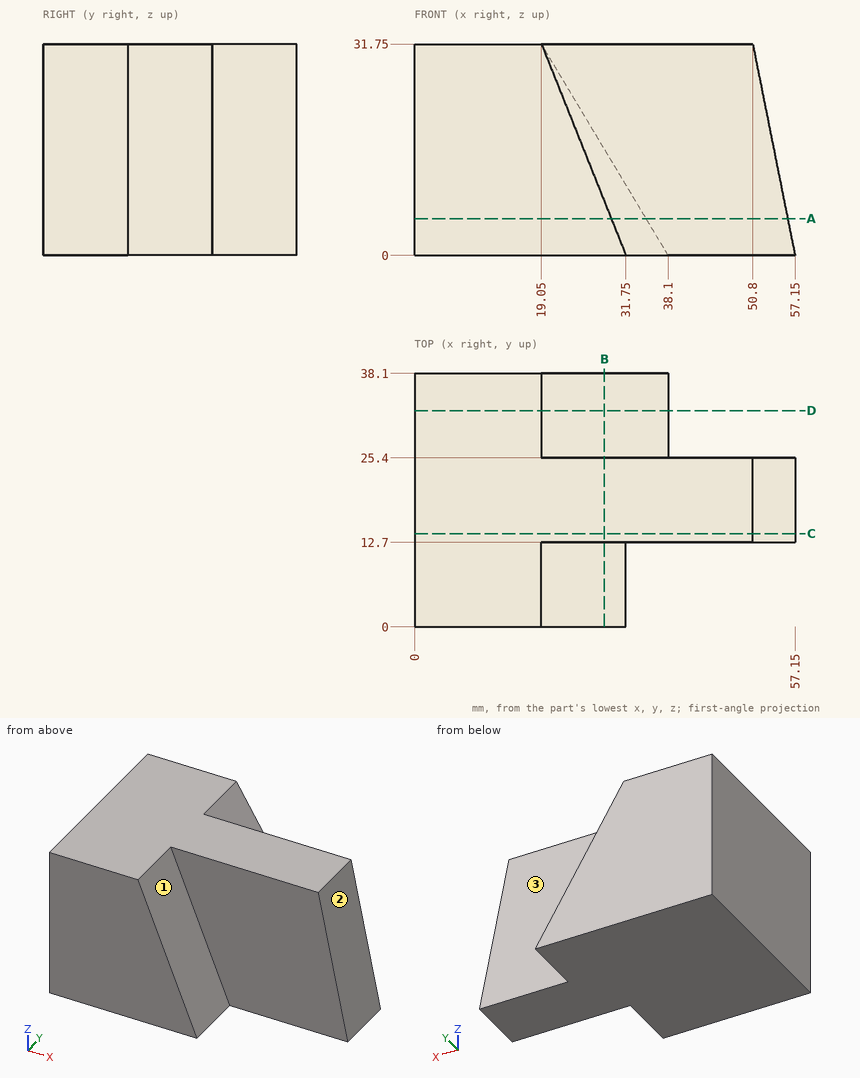
Print and shaded views of the part. All mm, measured from the part's lowest x, y and z. A direction names the side the tool comes from. Coordinates: 2 decimals unless noted, no trailing zeros. Order: outer loops, then holes, each group sorted by start corner. A loop starts at its lowest first (then second) coordinate and runs counter-clockwise, first axis right, second up.
(1) Pin check, flat tips, straight feed: pin 1 Ø9.5 at (x, z) = (39.5, 21.5) entering from -Y; pin 2 Ø4 at (y, z) = (29.5, 25) entering from +X. Stop position of each tip, or through.
Check sheet entries:
pin 1: stops at y = 12.7
pin 2: stops at x = 24.3
(2) Slice it at A-A, the plane z = 5.5. Write the cut outline in (x, y), and give its area (3 significant figures).
Check sheet entries:
outline: (0, 0) - (29.55, 0) - (29.55, 12.7) - (56.05, 12.7) - (56.05, 25.4) - (34.8, 25.4) - (34.8, 38.1) - (0, 38.1) - close
area: 1,530 mm2
(3) Tool access for the marked faces 1, 2 and 3: list every direction of +Z, -Z, +X, -X, +Y, -Y with a clear straight run to the whole face (end or side of a thin tool).
Check sheet entries:
face 1: +Z, +X, -Y
face 2: +Z, +X, +Y, -Y
face 3: +Z, +X, +Y
(4) Slice it at C-C, the plane y = 14. Write the cut outline in (x, z), and give its area (3 significant figures).
Check sheet entries:
outline: (0, 0) - (57.15, 0) - (50.8, 31.75) - (0, 31.75) - close
area: 1,710 mm2
(5) Probe L1, parallel to Y at x = 26.5, z = 28.5; L2, parallel to Y at x = 27.5, z = 13; L3, parallel to X at y = 3.5, z = 23.5. List the from-to ranges inside material, lowest first.
Check sheet entries:
L1: y = 12.7 to 25.4
L2: y = 12.7 to 38.1
L3: x = 0 to 22.35
(6) Slice it at B-B, the plane x = 28.5. Write the cut outline in (y, z) (3 decimals).
Check sheet entries:
outline: (0, 0) - (38.1, 0) - (38.1, 16) - (25.4, 16) - (25.4, 31.75) - (12.7, 31.75) - (12.7, 8.125) - (0, 8.125) - close
(7) Slice it at D-D, the plane y = 32.5. Write the cut outline in (x, z), and give its area (3 significant figures).
Check sheet entries:
outline: (0, 0) - (38.1, 0) - (19.05, 31.75) - (0, 31.75) - close
area: 907 mm2
